Here's how the part is built. I have some questions about the finished solid (model axes, mm). Round coordinates to 2 decimals unless told otherwise and drop trailing zeros. Loops run counter-clockwise (first coordinate to the right, second up) from the corner with the lowest first, then second, coordinate; pieces in that order, holes last. Notation, with made-up numbers: (56, 67) -> (109, 67) arc R15 ccw to (109, 71) -> close; hole circle Ø10 at (57, -27). An arc over 180 degrees is marked (long way). Use one line per item in the form item = value. Start each with the question number.
Item 1: If we section it at C-C (x = -3.5): Write out the boundary of the cut face in (y, z) (3 decimals), then the cut area to 3 significant figures.
Item 2: If I drill on L1, parallel to X at y = -8.25, z = 258 (3 decimals); L2, parallel to Y at x = 8.5, z = 19.5 (3 decimals), over which ranges is the centre line in solid material (lowest first)? Write a range as [from, to].
Item 3: If we section it at A-A (y = -6): Write out the boundary of the cut face in (x, z) (3 decimals), then the cut area to 3 significant figures.
Item 4: I'm going to push flat-ended pins straight in: pin 1 Ø6 at (x, z) = (2, 202) entering from -Y; pin 2 Ø5 at (x, z) = (-9, 175.5) entering from -Y (3 decimals); pin 3 Ø4 at (x, y) = (-6, 3) entering from -Z. Where does each tip first touch, or does it pass through?
Item 5: If we section it at B-B (z = 192.5): Write out the boundary of the cut face in (x, y) (3 decimals), then the cut area to 3 significant figures.
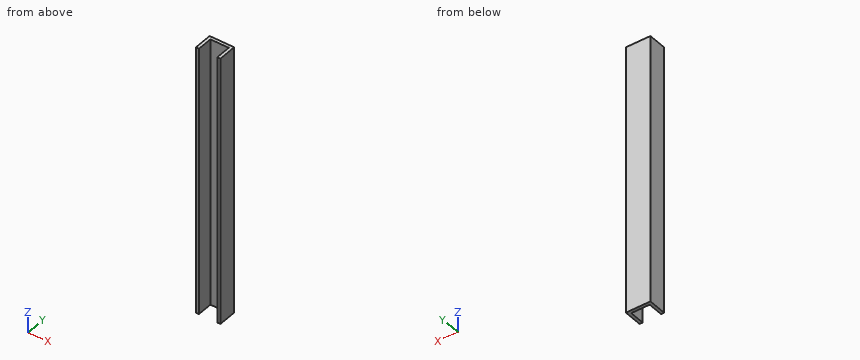
Autodesk Inventor part; units mm, degrees
ref_plane "YZ Plane" through (0, 0, 0) normal (1, 0, 0) x (0, 1, 0)
ref_plane "XZ Plane" through (0, 0, 0) normal (0, 1, 0) x (-1, 0, 0)
ref_plane "XY Plane" through (0, 0, 0) normal (0, 0, 1) x (1, 0, 0)
sketch "Sketch1" plane through (0, 0, 0) normal (0, 0, 1) x (1, 0, 0)
  line L0 (12.7, -9.525) -> (12.7, 9.525)
  line L1 (12.7, 9.525) -> (-12.7, 9.525)
  line L2 (-12.7, 9.525) -> (-12.7, -9.525)
  line L3 (-12.7, -9.525) -> (12.7, 9.525) construction
  line L4 (12.7, -9.525) -> (-12.7, 9.525) construction
  line L5 (9.525, -6.35) -> (9.525, 6.35)
  line L6 (9.525, 6.35) -> (-9.525, 6.35)
  line L7 (-9.525, 6.35) -> (-9.525, -6.35)
  line L8 (-9.525, -6.35) -> (9.525, 6.35) construction
  line L9 (9.525, -6.35) -> (-9.525, 6.35) construction
  line L10 (-9.525, -6.35) -> (-9.525, -9.525)
  line L11 (-9.525, -9.525) -> (-12.7, -9.525)
  line L12 (9.525, -6.35) -> (9.525, -9.525)
  line L13 (9.525, -9.525) -> (12.7, -9.525)
  point P0 (0, 0)
  dimension "d0" = 25.4
  dimension "d1" = 19.05
  dimension "d4" = 19.05
  dimension "d5" = 12.7
  dimension "d6" = 90
extrude "Extrusion2" add sketch "Sketch1" along normal blind 279.4
properties part number "case"
Values found:
q1.outline = (6.35, 0) -> (9.525, 0) -> (9.525, 279.4) -> (6.35, 279.4) -> close
q1.area = 887 mm2
q2.L1 = [-12.7, -9.525], [9.525, 12.7]
q2.L2 = [6.35, 9.525]
q3.outline = (-12.7, 0) -> (-9.525, 0) -> (-9.525, 279.4) -> (-12.7, 279.4) -> close; (9.525, 0) -> (12.7, 0) -> (12.7, 279.4) -> (9.525, 279.4) -> close
q3.area = 1,770 mm2
q4.pin_1 = 6.35
q4.pin_2 = -9.525
q4.pin_3 = through
q5.outline = (-12.7, -9.525) -> (-9.525, -9.525) -> (-9.525, 6.35) -> (9.525, 6.35) -> (9.525, -9.525) -> (12.7, -9.525) -> (12.7, 9.525) -> (-12.7, 9.525) -> close
q5.area = 181 mm2
